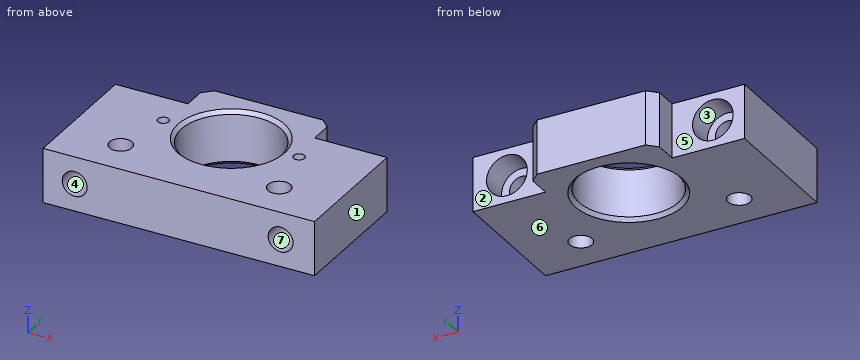
Autodesk Inventor part; units mm, degrees
ref_plane "YZ Plane" through (0, 0, 0) normal (1, 0, 0) x (0, 1, 0)
ref_plane "XZ Plane" through (0, 0, 0) normal (0, 1, 0) x (-1, 0, 0)
ref_plane "XY Plane" through (0, 0, 0) normal (0, 0, 1) x (1, 0, 0)
sketch "Sketch1" plane through (0, 0, 0) normal (0, 0, 1) x (1, 0, 0)
  line L0 (-30, 0) -> (30, 0)
  line L1 (30, 0) -> (30, 29)
  line L2 (30, 29) -> (14, 29)
  line L3 (14, 29) -> (14, 36)
  line L4 (14, 36) -> (-14, 36)
  line L5 (-14, 36) -> (-14, 29)
  line L6 (-14, 29) -> (-30, 29)
  line L7 (-30, 29) -> (-30, 0)
  point P0 (0, 0)
  point P1 (0, 0)
  dimension "d0" = 60
  dimension "d1" = 36
  dimension "d2" = 7
  dimension "d3" = 28
extrude "Extrusion1" add sketch "Sketch1" along normal mid plane 12
sketch "Sketch2" plane through (0, 0, 6) normal (0, 0, 1) x (1, 0, 0)
  line L0 (-30, 0) -> (30, 0)
  point P0 (0, 0)
  point P1 (0, 21)
  point P2 (0, 0)
  dimension "d6" = 21
hole "Hole1" at (0, 21, 6) direction (0, 0, -1) diameter 22 end through all
chamfer "Chamfer1" distance 0.8 angle 45 2 edges at (0, 32, 6) (0, 32, -6)
chamfer "Chamfer2" distance 2 angle 45 2 edges at (-14, 36, 0) (14, 36, 0)
sketch "Sketch3" plane through (-30, 29, 6) normal (0, 1, 0) x (1, 0, 0)
  line L0 (0, 12) -> (0, 0)
  line L1 (60, 12) -> (60, 0)
  point P0 (30, 6)
  point P1 (7, 6)
  point P2 (52.5, 6)
  dimension "d20" = 45.5
  dimension "d21" = 7
  dimension "d22" = 7.5
hole "Hole2" at (-23, 29, 0) at (22.5, 29, 0) direction (0, -1, 0) diameter 5.5 end through all counterbore diameter 9 counterbore depth 6
sketch "Sketch4" plane through (0, 0, 6) normal (0, 0, 1) x (1, 0, 0)
  line L0 (-30, 0) -> (30, 0)
  line L1 (-30, 29) -> (-30, 0)
  point P0 (0, 0)
  point P1 (-17.5, 8.5)
  point P2 (17.5, 8.5)
  dimension "d30" = 35
  dimension "d31" = 8.5
  dimension "d32" = 12.5
hole "Hole3" at (-17.5, 8.5, 6) at (17.5, 8.5, 6) direction (0, 0, -1) diameter 5 end through all
sketch "Sketch5" plane through (0, 0, 6) normal (0, 0, 1) x (1, 0, 0)
  circle A0 centre (0, 21) radius 11
  circle A1 centre (0, 21) radius 11
  point P0 (0, 0)
  point P1 (-15, 21)
  point P2 (15, 21)
  dimension "d40" = 30
  dimension "d41" = 15
hole "Hole4" at (-15, 21, 6) at (15, 21, 6) direction (0, 0, -1) diameter 2.459 depth 10 tip angle 118
properties part number "Lagerbock_Loslager" material "Aluminum 6061"
Work out the finished part from the listing and answer in its coordinate system (mm). Face numbers are marked on the shaded views. A direction names the side the tool comes from. Give positions to 0.01 mm unless a question says otherwise; leave off trailing zeros. Order: outer loops, then holes, each group sorted by start corner. A loop starts at its lowest first (then second) coordinate and runs counter-clockwise, first axis right, second up.
1. Straight lines are drawn through the part: L1, parallel to X at y = 16.75, z = 0; L2, parallel to Z at x = -23, y = 8; L3, parallel to X at y = 21, z = 2.25. For each, find the intervals that lie inside material, in ascending order.
Result sheet:
L1: x = -30 to -25.75, -20.25 to -10.15, 10.15 to 19.75, 25.25 to 30
L2: z = -6 to -2.75, 2.75 to 6
L3: x = -30 to -24.58, -21.42 to -16.23, -13.77 to -11, 11 to 13.77, 16.23 to 20.92, 24.08 to 30
2. Section C-C, the plane y = 12 is taken. Give the number of separate pieces and of enclosed holes in the cut face, and give its area (3 significant figures).
Result sheet:
separate pieces: 2
enclosed holes: 2
area: 519 mm2
3. Section D-D, the plane x = -17.5 is taken. Determine the outline of the cut face in (y, z), and give its area (3 significant figures).
Result sheet:
outline: (0, -6) - (6, -6) - (6, 6) - (0, 6) - close; (11, -6) - (29, -6) - (29, 6) - (11, 6) - close
area: 288 mm2
4. Section A-A, the plane x = 0 is taken. Determine the outline of the cut face in (y, z).
Result sheet:
outline: (0, -6) - (9.2, -6) - (10, -5.2) - (10, 5.2) - (9.2, 6) - (0, 6) - close; (32, -5.2) - (32.8, -6) - (36, -6) - (36, 6) - (32.8, 6) - (32, 5.2) - close
5. The mould has two halves that part along Z. Classify the marked faces 4, 5, 6 and 7: released by +Z, released by -Z, zero draft, split by the parting line, or undercut.
Result sheet:
face 4: undercut
face 5: zero draft
face 6: released by -Z
face 7: undercut
6. Section B-B, the plane x = 22.5 is taken. Determine the outline of the cut face in (y, z).
Result sheet:
outline: (0, -6) - (29, -6) - (29, -4.5) - (23, -4.5) - (23, -2.75) - (0, -2.75) - close; (0, 2.75) - (23, 2.75) - (23, 4.5) - (29, 4.5) - (29, 6) - (0, 6) - close
7. Each of these flat-tipped pins is pushed along its axis until it touches: P1, Ø20, axis at x = 0, y = 21, coming from the +Z side; P2, Ø1.5, axis at y = 31.5, z = 2, coming from the -X side; P3, Ø3, axis at x = 16.5, z = -4.5, coming from the -Y side; P4, Ø2, axis at x = -15, y = 21, coming from the +Z side. Where does it stop, or does it pass through?
Result sheet:
P1: passes through
P2: stops at x = -14
P3: stops at y = 0
P4: stops at z = -4.14
8. For the marked faces 1, 2 and 3, determine the directions among +Z, -Z, +X, -X, +Y, -Y from which every point of the face is accessible in a straight line to the end or side of a thin tool.
Result sheet:
face 1: +Z, -Z, +X, +Y, -Y
face 2: +Z, -Z, +X, +Y
face 3: +Y
